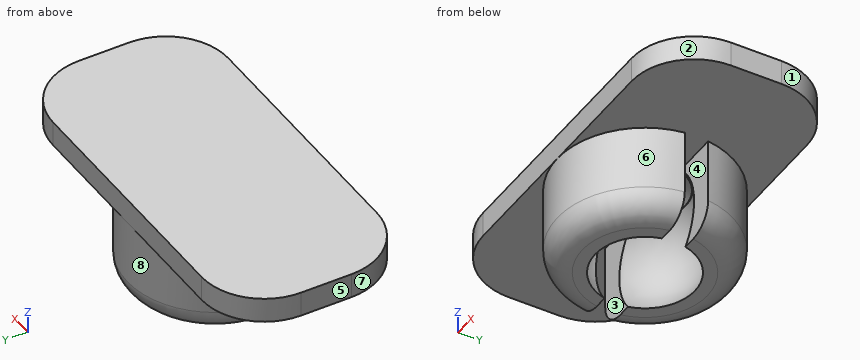
Autodesk Inventor part; units mm, degrees
ref_plane "YZ Plane" through (0, 0, 0) normal (1, 0, 0) x (0, 1, 0)
ref_plane "XZ Plane" through (0, 0, 0) normal (0, 1, 0) x (-1, 0, 0)
ref_plane "XY Plane" through (0, 0, 0) normal (0, 0, 1) x (1, 0, 0)
sketch "Sketch1" plane through (0, 0, 0) normal (0, 0, 1) x (1, 0, 0)
  line L0 (5, 0) -> (25, 0)
  line L1 (30, -5) -> (30, -9)
  line L2 (25, -14) -> (5, -14)
  line L3 (0, -9) -> (0, -5)
  arc A0 (0, -9) -> (5, -14) centre (5, -9) ccw
  arc A1 (5, 0) -> (0, -5) centre (5, -5) ccw
  arc A2 (30, -5) -> (25, 0) centre (25, -5) ccw
  arc A3 (25, -14) -> (30, -9) centre (25, -9) ccw
  point P0 (0, 0)
  point P1 (30, -14)
  point P2 (30, 0)
  point P3 (0, -14)
  dimension "d0" = 30
  dimension "d1" = 14
  dimension "d2" = 5
extrude "Extrusion1" add sketch "Sketch1" along normal blind 2
ref_plane "Work Plane1" through (15, -9, 0) normal (-1, 0, 0) x (0, 0, 1)
sketch "Sketch2" plane through (15, -9, 0) normal (-1, 0, 0) x (0, 0, 1)
  circle A0 centre (-3.9426, 2) radius 4.775 construction
  line L0 (-3.9426, 2) -> (0, 2) construction
  line L1 (0, 0) -> (0, 4) construction
  line L2 (0, 4) -> (0, 9) construction
  line L3 (0, 9) -> (-5.1622, 9) construction
  line L4 (-7.1622, 7) -> (-7.1622, 5.2744) construction
  line L5 (-7.1622, 5.2744) -> (0, 5.2744) construction
  line L6 (0, 5.2744) -> (0, 9) construction
  arc A1 (0, 5.2744) -> (-7.1622, 5.9874) centre (-3.9426, 2) ccw
  line L7 (-7.1622, 5.9874) -> (-7.1622, 7)
  line L8 (-5.1622, 9) -> (0, 9)
  line L9 (0, 9) -> (2, 9)
  line L10 (0, 9) -> (0, 5.2744)
  arc A2 (-5.1622, 9) -> (-7.1622, 7) centre (-5.1622, 7) ccw
  line L11 (-5.1622, 9) -> (0, 9)
  dimension "d5" = 9.55
  dimension "d6" = 5.125
  dimension "d7" = 2
revolve "Revolution1" add sketch "Sketch2" angle 360 about axis through (15, -7, -3.9426) along (0, 0, 1)
sketch "Sketch3" plane through (15, -9, 0) normal (-1, 0, 0) x (0, 0, 1)
  line L0 (0, 0) -> (0, 4)
  line L1 (-7.1622, -1.9874) -> (-7.1622, 5.9874)
  line L2 (0, 2) -> (-7.1622, 2)
  line L3 (-7.1622, 2) -> (-7.1622, 2.9338)
  line L4 (-7.1622, 2.9338) -> (0, 2.9338)
  line L5 (0, 2.9338) -> (0, 2)
  line L6 (-7.1622, 2) -> (0, 2)
  line L7 (0, 2) -> (0, 1.066)
  line L8 (0, 1.066) -> (-7.1622, 1.066)
  line L9 (-7.1622, 1.066) -> (-7.1622, 2)
  point P0 (0, 9)
  point P1 (0, 2.9338)
  point P2 (-7.1622, 1.066)
  dimension "d9" = 0.934
extrude "Extrusion2" cut sketch "Sketch3" along normal through all both and the other way through all
sketch "Sketch4" plane through (15, -9, 0) normal (-1, 0, 0) x (0, 0, 1)
  line L0 (0, 4) -> (0, 9)
  arc A0 (1.1539, 2) -> (0, 5.2289) centre (-3.9407, 2) ccw
  line L1 (0, 4) -> (0, 0)
  line L2 (0, 2) -> (0, 5.2289)
  line L3 (0, 2) -> (1.1539, 2)
revolve "Revolution2" cut sketch "Sketch4" angle 360 about axis through (15, -7, -3.9426) along (0, 0, 1)
properties part number "Wheelmount"
Could you check a few things on this model? Use its own coordinates, in mm. Face numbers are marked on the shaded views. A direction names the side the tool comes from. Round coordinates to 2 decimals unless told otherwise and drop trailing zeros. Order: outer loops, then holes, each group sorted by start corner. A loop starts at its lowest first (then second) coordinate and runs counter-clockwise, first axis right, second up.
(1) Which directions (+Z, -Z, +X, -X, +Y, -Y) give clear straight access to the entire face, cutting with the end or side of a thin tool? Please do the marked faces 4, 5, 6, 7 and 8.
Response values:
face 4: -Z, +X, -X
face 5: +Z, -Z, -X, +Y, -Y
face 6: -Z, -Y
face 7: +Z, -Z, -X, -Y
face 8: -Z, +Y
(2) Please list where these lines run through material, in increasing order: line 1 along Z through (x, y) = (4, -6.5); line 2 along Y through (x, z) = (8.75, -1.75); line 3 along X through (y, z) = (-4.75, -6.25).
Response values:
line 1: z = 0 to 2
line 2: y = -10.15 to -7.93, -6.07 to -3.85
line 3: x = 8.71 to 11.02, 18.98 to 21.29
(3) Imagine slicing it at C-C (x = 26.25). Write out the boundary of the cut face in (y, z).
Response values:
outline: (-13.84, 0) - (-0.16, 0) - (-0.16, 2) - (-13.84, 2) - close
(4) Imagine slicing it at B-B (x = 6.75). Write out the boundary of the cut face in (y, z), plus the area to 3 significant figures.
Response values:
outline: (-14, 0) - (0, 0) - (0, 2) - (-14, 2) - close
area: 28.0 mm2
(5) I'm going to push flat-ended pins straight in: pin 1 (1.9 mm diameter, centred on x = 21, z = -2.5, fed in from -Y); pin 2 (4 mm diameter, centred on y = -12.5, z = -0.5, fed in from +X); pin 3 (5 mm diameter, centred on x = 16, y = -4.5, fed in from -Z); pin 4 (3 mm diameter, centred on x = 21, z = -4.5, fed in from +Y). Where does each tip first touch, or does it pass through?
Response values:
pin 1: stops at y = -11.85
pin 2: stops at x = 29.75
pin 3: stops at z = -7.16
pin 4: stops at y = -1.64
(6) Imagine slicing it at A-A (z = 1.5). Write out the boundary of the cut face in (x, y), plus the area to 3 significant figures.
Response values:
outline: (0, -9) arc R5 ccw to (5, -14) - (25, -14) arc R5 ccw to (30, -9) - (30, -5) arc R5 ccw to (25, 0) - (5, 0) arc R5 ccw to (0, -5) - close
area: 399 mm2
(7) If we mould it in two halves opening along Y, with no side actions, what happens to the marked faces 1, 2 and 3? For each: released by +Y, released by -Y, zero draft, split by the parting line, or undercut.
Response values:
face 1: released by +Y
face 2: released by -Y
face 3: undercut
